```python
from build123d import *

# Parameters (mm, degrees)
PAD_DEPTH       = 50
SKETCH001_R     = 4
POCKET_DEPTH    = 15.001
POCKET001_DEPTH = 7


with BuildPart() as part:
    # Sketch → Pad (new body)
    with BuildSketch(Plane.YZ):
        with BuildLine():
            Line((0, 0), (20, 0))
            Line((20, 0), (20, 12))
            ThreePointArc((20, 12), (19.12132, 14.12132), (17, 15))
            Line((3, 15), (17, 15))
            ThreePointArc((3, 15), (0.87868, 14.12132), (0, 12))
            Line((0, 0), (0, 12))
        make_face()
    extrude(amount=PAD_DEPTH)

    # Sketch001 → Pocket (cut, through all)
    with BuildSketch(Plane(origin=(0, 0, 15), x_dir=(0, -1, 0), z_dir=(0, 0, 1))):
        with Locations((-10, 40)):
            Circle(SKETCH001_R)
        with Locations((-10, 10)):
            Circle(SKETCH001_R)
    extrude(amount=-POCKET_DEPTH, mode=Mode.SUBTRACT)

    # Sketch002 → Pocket001 (cut)
    with BuildSketch(Plane(origin=(0, 0, 15), x_dir=(0, -1, 0), z_dir=(0, 0, 1))):
        Polygon((-16.226723, 36.405), (-10, 32.81), (-3.773277, 36.405), (-3.773277, 43.595), (-10, 47.19), (-16.226723, 43.595), align=None)
        Polygon((-16.226723, 6.405), (-10, 2.81), (-3.773277, 6.405), (-3.773277, 13.595), (-10, 17.19), (-16.226723, 13.595), align=None)
    extrude(amount=-POCKET001_DEPTH, mode=Mode.SUBTRACT)


solid = part.part
```
Input: part model. Units: mm. Frame: model coordinates. A direction names the side the tool comes from. Give positions to 0.01 mm unless a question says otherwise; leave off trailing zeros. Loops run counter-clockwise (first coordinate to the right, second up) from the corner with the lowest first, then second, coordinate; pieces in that order, holes last.
1) Mould query, pull axis X, two halves, no side actions, for faces 1 (the cylindrical face through (24.65, 0.9, 14.14)), 2 (the flat face through (15.4, 13.1, 11.5)), 3 (the flat face through (0, 10, 8)). Classes: released by +X, released by -X, zero draft, split by the parting line, or undercut.
A:
face 1: zero draft
face 2: undercut
face 3: released by -X
2) Section query C-C on z = 4. Return the cut outline in (x, y).
A:
outline: (0, 0) - (50, 0) - (50, 20) - (0, 20) - close; hole circle Ø8 at (10, 10); hole circle Ø8 at (40, 10)
3) Line query: L1, parallel to X at y = 10.25, z = 5.5; L2, parallel to X at y = 10, z = 9; L3, parallel to Y at x = 42, z = 10. Output: solid intervals per line, ascending.
A:
L1: x = 0 to 6.01, 13.99 to 36.01, 43.99 to 50
L2: x = 0 to 2.81, 17.19 to 32.81, 47.19 to 50
L3: y = 0 to 3.77, 16.23 to 20
4) Section query A-A on x = 40. Return the cut outline in (y, z), and give its area (3 significant figures).
A:
outline: (0, 0) - (6, 0) - (6, 8) - (3.77, 8) - (3.77, 15) - (3, 15) arc R3 ccw to (0, 12) - close; (14, 0) - (20, 0) - (20, 12) arc R3 ccw to (17, 15) - (16.23, 15) - (16.23, 8) - (14, 8) - close
area: 145 mm2
5) Reachability of faces 4 (the flat face through (25, 20, 6)), 5 (the flat face through (40, 16.227, 12)) from +Z, -Z, +X, -X, +Y, -Y: full face, straight path, thin tool, end or side. Return the list, or none.
A:
face 4: +Z, -Z, +X, -X, +Y
face 5: +Z
6) Section query B-B on z = 11.25. Return the cut outline in (x, y) (3 decimals).
A:
outline: (0, 0) - (50, 0) - (50, 20) - (0, 20) - close; hole (2.81, 10) - (6.405, 3.773) - (13.595, 3.773) - (17.19, 10) - (13.595, 16.227) - (6.405, 16.227) - close; hole (32.81, 10) - (36.405, 3.773) - (43.595, 3.773) - (47.19, 10) - (43.595, 16.227) - (36.405, 16.227) - close
7) Contact query for a flat-ended pin moving along its axis: pin 1 (10.5 mm diameter, centred on x = 10, y = 10, fed in from +Z). Output: stop coordinate, or through.
A:
pin 1: stops at z = 8
